```python
from build123d import *

# Parameters (mm, degrees)
SKETCH1_W           = 185.1152
SKETCH1_H           = 115.7478
BOSS_EXTRUDE1_DEPTH = 5.08
BOSS_EXTRUDE2_DEPTH = 7.62


with BuildPart() as part:
    # Sketch1 → Boss-Extrude1 (new body)
    with BuildSketch(Plane(origin=(0, 0, 0), x_dir=(1, 0, 0), z_dir=(0, 1, 0))):
        with Locations((92.5576, 57.8739)):
            Rectangle(SKETCH1_W, SKETCH1_H)
    extrude(amount=BOSS_EXTRUDE1_DEPTH)

    # Sketch2 → Boss-Extrude2 (add)
    with BuildSketch(Plane(origin=(0, 5.08, 0), x_dir=(1, 0, 0), z_dir=(0, 1, 0))):
        Polygon((2.8321, 112.9284), (182.2831, 112.9284), (182.2831, 2.8194), (104.4321, 2.8194), (104.4321, 58.3184), (60.7441, 58.3184), (60.7441, 2.8194), (2.8321, 2.8194), align=None)
        Polygon((4.6101, 111.1504), (4.6101, 4.5974), (58.9661, 4.5974), (58.9661, 60.0964), (106.2101, 60.0964), (106.2101, 4.5974), (180.5051, 4.5974), (180.5051, 111.1504), align=None, mode=Mode.SUBTRACT)
    extrude(amount=BOSS_EXTRUDE2_DEPTH)


solid = part.part
```
Model file for the job. Use its own axes, mm. A direction names the side the tool comes from. Coordinates: 2 decimals unless noted, no trailing zeros. Loops run counter-clockwise (first coordinate to the right, second up) from the corner with the lowest first, then second, coordinate; pieces in that order, holes last. Notation, with made-up numbers: (-40, -35) - (10, -35) arc R26 ccw to (10, 0) - close; hole circle Ø1 at (70, -35.75). An arc over 180 degrees is marked (long way). Write item = value, one per line. Start each with the question number.
Item 1: Wall check: probe 1 along X at (y, z) = (7, -36); probe 2 along X at (y, z) = (7.5, -4.5); probe 3 along Z at (x, y) = (173, 11.5). Give the ranges that are in metal, low to high. Write a range as [from, to].
Item 2: Saw through at D-D, the plane z = -18. List the corners of the cut face in (x, y).
Item 3: Drop flat-ended pins along their axis: pin 1 Ø8 at (x, z) = (90, -85.5) entering from +Y; pin 2 Ø6 at (y, z) = (10.5, -55) entering from +X; pin 3 Ø2.5 at (y, z) = (9, -29.5) entering from -X; pin 4 Ø3 at (x, y) = (30.5, 3) entering from +Z. Give the stop position or say it passes through.
Item 4: Pull direction X, two halves, no side cores. Call faces 1 (the face through (0, 3, -57)), 2 (the face through (60, 12.7, -34)), 3 (the face through (106.21, 9, -33)): +X half, -X half, draft (parallel to the pull), parting line (faces both ways), or undercut.
Item 5: Saw through at C-C, the plane x = 116. List the corners of the cut face in (y, z).
Item 6: 3-axis set-ups, long thin cutter, end or side, ignore diameter. For faces 4 (the face through (4.61, 9, -59)), 5 (the face through (2.832, 9, -57)), 6 (the face through (144, 9, -2.819)): which of +Z, -Z, +X, -X, +Y, -Y reach the whole face in a straight line?
Item 7: Saw through at B-B, the plane z = -70.5. List the corners of the cut face in (x, y).
Item 8: Saw through at A-A, the plane y = 9.25. List the corners of the cut face in (x, z), then the cut area to 3 significant figures.
Answers:
q1.probe_1 = [2.83, 4.61], [58.97, 60.74], [104.43, 106.21], [180.51, 182.28]
q1.probe_2 = [2.83, 60.74], [104.43, 182.28]
q1.probe_3 = [-112.93, -111.15], [-4.6, -2.82]
q2.outline = (0, 0) - (185.12, 0) - (185.12, 5.08) - (182.28, 5.08) - (182.28, 12.7) - (180.51, 12.7) - (180.51, 5.08) - (106.21, 5.08) - (106.21, 12.7) - (104.43, 12.7) - (104.43, 5.08) - (60.74, 5.08) - (60.74, 12.7) - (58.97, 12.7) - (58.97, 5.08) - (4.61, 5.08) - (4.61, 12.7) - (2.83, 12.7) - (2.83, 5.08) - (0, 5.08) - close
q3.pin_1 = 5.08
q3.pin_2 = 182.28
q3.pin_3 = 2.83
q3.pin_4 = 0
q4.face_1 = -X half
q4.face_2 = draft
q4.face_3 = undercut
q5.outline = (0, -115.75) - (5.08, -115.75) - (5.08, -112.93) - (12.7, -112.93) - (12.7, -111.15) - (5.08, -111.15) - (5.08, -4.6) - (12.7, -4.6) - (12.7, -2.82) - (5.08, -2.82) - (5.08, 0) - (0, 0) - close
q6.face_4 = +Y
q6.face_5 = +Z, -Z, -X, +Y
q6.face_6 = +Z, +X, -X, +Y
q7.outline = (0, 0) - (185.12, 0) - (185.12, 5.08) - (182.28, 5.08) - (182.28, 12.7) - (180.51, 12.7) - (180.51, 5.08) - (4.61, 5.08) - (4.61, 12.7) - (2.83, 12.7) - (2.83, 5.08) - (0, 5.08) - close
q8.outline = (2.83, -112.93) - (182.28, -112.93) - (182.28, -2.82) - (104.43, -2.82) - (104.43, -58.32) - (60.74, -58.32) - (60.74, -2.82) - (2.83, -2.82) - close; hole (4.61, -111.15) - (180.51, -111.15) - (180.51, -4.6) - (106.21, -4.6) - (106.21, -60.1) - (58.97, -60.1) - (58.97, -4.6) - (4.61, -4.6) - close
q8.area = 1,210 mm2
